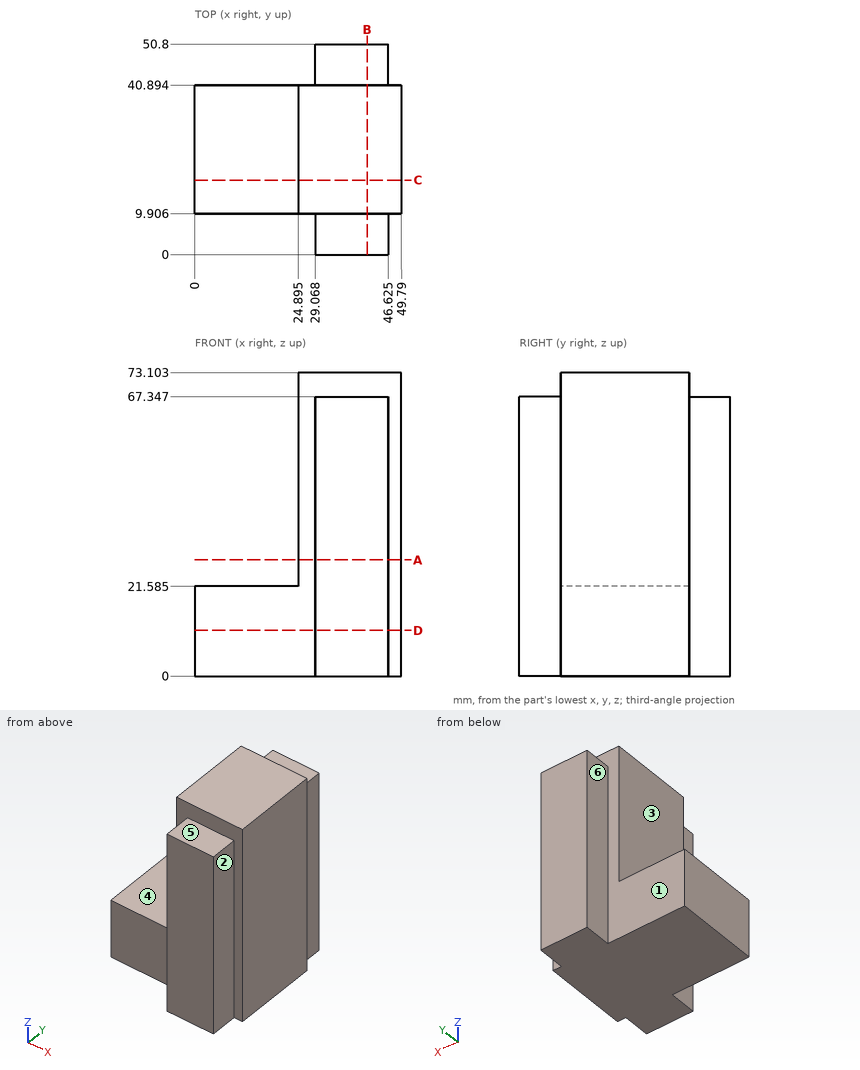
Geometry: see drawing. Coordinates: mm, zero at the bounding-box minimum. A direction names the side the tool comes from. Coordinates: 2 decimals unless noted, no trailing zeros. Loops run counter-clockwise (first coordinate to the right, second up) from the corner with the lowest first, then second, coordinate; pieces in that order, holes last. Notation, with made-up numbers: (55, 28) - (66, 28) arc R26 cw to (66, 47) - close; hole circle Ø1 at (-32.5, -37.5). An arc over 180 degrees is marked (long way). Answer in a Markdown table with one row per item.
(1) Pin query (flat end, axial travel): P1, Ø10, axis at x = 6, y = 19.5, coming from the +Z side (1 decimal); P2, Ø11, axis at x = 36, y = 6.5, coming from the +Z side; P3, Ø25, axis at x = 16.5, z = 47.5, coming from the -Y side; P4, Ø8, axis at y = 46, z = 20.5, coming from the -X side. Return the tip coordinate at first contact, or that it passes through.
Model answer:
| item | result |
|---|---|
| P1 | stops at z = 21.6 |
| P2 | stops at z = 73.1 |
| P3 | stops at y = 9.91 |
| P4 | stops at x = 29.07 |
(2) Mould query, pull axis X, two halves, no side actions, for the marked faces 1, 2 and 3. Classes: pulls with the +X half, pulls with the -X half, needs draft (parallel to the pull), parting line crosses it, or undercut.
Model answer:
| item | result |
|---|---|
| face 1 | needs draft |
| face 2 | pulls with the +X half |
| face 3 | pulls with the -X half |
(3) Cut plane B-B on x = 41.5. Output: boundary loops of the cut face in (y, z).
Model answer:
| item | result |
|---|---|
| outline | (0, 0) - (50.8, 0) - (50.8, 67.35) - (40.89, 67.35) - (40.89, 73.1) - (9.91, 73.1) - (9.91, 67.35) - (0, 67.35) - close |
(4) Cut plane C-C on y = 18. Output: boundary loops of the cut face in (x, z) (1 decimal), plus the area to 3 significant figures.
Model answer:
| item | result |
|---|---|
| outline | (0, 0) - (49.8, 0) - (49.8, 73.1) - (24.9, 73.1) - (24.9, 21.6) - (0, 21.6) - close |
| area | 2,360 mm² |
(5) Material intervals for L1, parallel to Z at x = 40, y = 45; L2, parallel to X at y = 34, z = 47.5 (1 decimal); L3, parallel to Y at x = 28.5, z = 23, sorted ascending. Write a range as from..to.
Model answer:
| item | result |
|---|---|
| L1 | z = 0..67.35 |
| L2 | x = 24.9..49.8 |
| L3 | y = 9.91..40.89 |
(6) Set-up query: the marked faces 4, 5 and 6. Return all of +Z, -Z, +X, -X, +Y, -Y with unobstructed straight access to the full face (end or side cutting, diameter ignored); none if empty.
Model answer:
| item | result |
|---|---|
| face 4 | +Z, -X, +Y, -Y |
| face 5 | +Z, +X, -X, -Y |
| face 6 | +Z, -Z, -X, +Y |
(7) Cut plane A-A on z = 28. Output: boundary loops of the cut face in (x, y) (1 decimal), plus the area to 3 significant figures.
Model answer:
| item | result |
|---|---|
| outline | (24.9, 9.9) - (29.1, 9.9) - (29.1, 0) - (46.6, 0) - (46.6, 9.9) - (49.8, 9.9) - (49.8, 40.9) - (46.6, 40.9) - (46.6, 50.8) - (29.1, 50.8) - (29.1, 40.9) - (24.9, 40.9) - close |
| area | 1,120 mm² |
(8) Cut plane D-D on z = 11. Output: boundary loops of the cut face in (x, y) (1 decimal).
Model answer:
| item | result |
|---|---|
| outline | (0, 9.9) - (29.1, 9.9) - (29.1, 0) - (46.6, 0) - (46.6, 9.9) - (49.8, 9.9) - (49.8, 40.9) - (46.6, 40.9) - (46.6, 50.8) - (29.1, 50.8) - (29.1, 40.9) - (0, 40.9) - close |
